The model under review builds one solid part; all positions refer to its coordinate system, in mm. Face numbers are marked on the shaded views. A direction names the side the tool comes from. Coordinates: 2 decimals unless noted, no trailing zeros. Order: outer loops, then holes, each group sorted by start corner. A loop starts at its lowest first (then second) coordinate and runs counter-clockwise, first axis right, second up. Notation, with made-up numbers: M 9,58.5 L 66,58.5 A31 ccw 66,93.5 Z; hole C -14,25 d8. An arc over 180 degrees is marked long. Answer in a Markdown table with one row per item.
Autodesk Inventor part; units mm, degrees
ref_plane "YZ Plane" through (0, 0, 0) normal (1, 0, 0) x (0, 1, 0)
ref_plane "XZ Plane" through (0, 0, 0) normal (0, 1, 0) x (-1, 0, 0)
ref_plane "XY Plane" through (0, 0, 0) normal (0, 0, 1) x (1, 0, 0)
sketch "Sketch2" plane through (0, 0, 0) normal (0, 1, 0) x (-1, 0, 0)
  line L0 (0, 0) -> (0, -12)
  line L1 (0, 0) -> (0, 10)
  line L2 (0, -12) -> (-2, -12)
  line L3 (-2, -12) -> (-2, -4)
  line L4 (-3, -4) -> (-2, -4)
  line L5 (-3, -4) -> (-3, -2.5) construction
  line L6 (-2, 10) -> (0, 10)
  line L7 (-3, -2.5) -> (0, -2.5) construction
  circle A0 centre (-1.2, -2.5) radius 0.95
  line L8 (-3, -4) -> (-3, 10)
  line L9 (-3, 10) -> (-2, 10)
  line L10 (0, 0) -> (-3, 0) construction
  dimension "d1" = 10
  dimension "d2" = 2
  dimension "d9" = 1.9
  dimension "d10" = 8
  dimension "d11" = 3
  dimension "d12" = 1.8
  dimension "d38" = 4
extrude "Extrusion1" add sketch "Sketch2" along normal blind 3.5
sketch "Sketch3" plane through (3, 0, 10) normal (1, 0, 0) x (0, 0, -1)
  line L0 (0, 0) -> (0, 3.5)
  line L1 (0, 1.75) -> (22, 1.75) construction
  line L2 (22, 1.75) -> (22, 2.15)
  line L3 (22, 0) -> (22, 3.5)
  line L4 (11, 2.15) -> (11, 1.35)
  line L5 (22, 2.15) -> (21.1843, 2.15)
  line L6 (18.8157, 2.15) -> (11, 2.15)
  line L7 (11, 1.35) -> (18.8157, 1.35)
  line L8 (21.1843, 1.35) -> (22, 1.35)
  arc A0 (18.8157, 1.35) -> (21.1843, 1.35) centre (20, 1.75) ccw
  arc A1 (21.1843, 2.15) -> (18.8157, 2.15) centre (20, 1.75) ccw
  line L9 (22, 1.75) -> (22, 1.35)
  point P0 (10, 0)
  dimension "d16" = 2
  dimension "d17" = 0.4
  dimension "d18" = 11
  dimension "d19" = 0.8
extrude "Extrusion2" cut sketch "Sketch3" against normal blind 10
sketch "Sketch4" plane through (0, 0, -12) normal (-1, 0, 0) x (0, 0, 1)
  point P0 (12, 0)
sketch "Sketch5" plane through (0, 0, -12) normal (-1, 0, 0) x (0, 0, 1)
  line L0 (16, 0) -> (16, -1)
  line L1 (16, -1) -> (22, -1)
  line L2 (22, 0) -> (16, 0)
  line L3 (16, 3.5) -> (16, 4.5)
  line L4 (16, 4.5) -> (22, 4.5)
  line L5 (22, 3.5) -> (16, 3.5)
  line L6 (22, 4.5) -> (27, 4.5)
  line L7 (27, 4.5) -> (27, -1)
  line L8 (27, -1) -> (22, -1)
  line L9 (22, 3.5) -> (22, 0)
  line L10 (12, 0) -> (12, 3.5) construction
  dimension "d23" = 1
  dimension "d24" = 1
  dimension "d27" = 5
  dimension "d39" = 5.5
  dimension "d40" = 4
extrude "Extrusion3" add sketch "Sketch5" against normal blind 3
sketch "Sketch6" plane through (0, 0, -12) normal (-1, 0, 0) x (0, 0, 1)
  line L0 (22, 1.75) -> (14, 1.75) construction
  line L1 (27, 4.5) -> (16, 4.5)
  circle A0 centre (24.5, 1.75) radius 0.95
  line L2 (27, -1) -> (27, 4.5)
  circle A1 centre (18.5, 1.75) radius 0.95
  point P0 (12, 0)
  dimension "d28" = 2.75
  dimension "d32" = 1.9
  dimension "d33" = 2.5
  dimension "d34" = 1.9
  dimension "d35" = 6
extrude "Extrusion4" cut sketch "Sketch6" against normal blind 3
properties part number "ferrule holder"
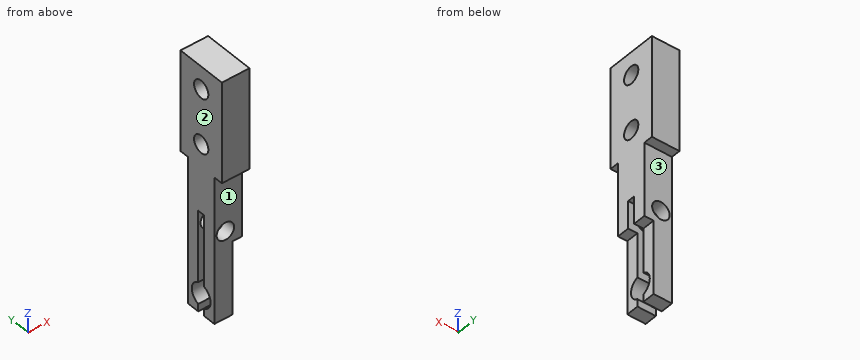
(1) Take a section at C-C (x = 2.6). Write out the cut boundary in (y, z), then the cut area to 3 significant figures.
Report:
| item | result |
|---|---|
| outline | M -1,4 L 0,4 L 0,-4 L 1.35,-4 L 1.35,-1 L 2.15,-1 L 2.15,-4 L 3.5,-4 L 3.5,4 L 4.5,4 L 4.5,15 L -1,15 Z; hole C 1.75,6.5 d1.9; hole C 1.75,12.5 d1.9 |
| area | 80.4 mm^2 |
(2) Take a section at A-A (x = 1.2). Write out the cut boundary in (y, z).
Report:
| item | result |
|---|---|
| outline | M -1,4 L 0,4 L 0,-1.55 L 1.35,-1.55 L 1.35,-1 L 2.15,-1 L 2.15,-1.55 L 3.5,-1.55 L 3.5,4 L 4.5,4 L 4.5,15 L -1,15 Z; M 0,-12 L 1.35,-12 L 1.35,-11.18 A1.25 cw 1.35,-8.82 L 1.35,-3.45 L 0,-3.45 Z; M 2.15,-12 L 3.5,-12 L 3.5,-3.45 L 2.15,-3.45 L 2.15,-8.82 A1.25 cw 2.15,-11.18 Z; hole C 1.75,6.5 d1.9; hole C 1.75,12.5 d1.9 |
(3) Take a section at B-B (z = -2.5). Write out the cut boundary in (x, y).
Report:
| item | result |
|---|---|
| outline | M 0,0 L 0.25,0 L 0.25,1.35 L 0,1.35 Z; M 0,2.15 L 0.25,2.15 L 0.25,3.5 L 0,3.5 Z; M 2.15,0 L 3,0 L 3,1.35 L 2.15,1.35 Z; M 2.15,2.15 L 3,2.15 L 3,3.5 L 2.15,3.5 Z |
(4) To check wall thickness, follow line 1 (Y direction, x = 0.8, z = 12.5); line 2 (Z direction, x = 1.2, y = 2.8); line 3 (Z direction, x = 1.9, y = 2.5). State the ranges of each line that lie inside material, in increasing order. Write a range as [from, to].
Report:
| item | result |
|---|---|
| line 1 | [-1, 0.8], [2.7, 4.5] |
| line 2 | [-12, -10.68], [-9.32, -3.45], [-1.55, 15] |
| line 3 | [-12, -11], [-9, -3.14], [-1.86, 5.92], [7.08, 11.92], [13.08, 15] |
(5) Take a section at D-D (y = 1.75). Write out the cut boundary in (x, z).
Report:
| item | result |
|---|---|
| outline | M 0,-1 L 3,-1 L 3,5.55 L 0,5.55 Z; M 0,7.45 L 3,7.45 L 3,11.55 L 0,11.55 Z; M 0,13.45 L 3,13.45 L 3,15 L 0,15 Z |
(6) Insertion check: P1, Ø0.5, axis at x = 1, y = 4, coming from the -Z side; P2, Ø0.9, axis at x = 1, z = -11.5, coming from the +Y side; P3, Ø0.7, axis at y = 3, z = -7.5, coming from the +X side. Each pin has a flat end and moves straight along its axis. Give the tip position at first contact, or say it passes through.
Report:
| item | result |
|---|---|
| P1 | z = 4 |
| P2 | y = 3.5 |
| P3 | x = 2 |
(7) Machinability: for the marked faces 1, 2 and 3, which of the approach directions +Z, -Z, +X, -X, +Y, -Y give a long, thin tool a straight path to every point of the face, cutting with its end or side? Answer none if there is none.
Report:
| item | result |
|---|---|
| face 1 | -Z, +X, -X, -Y |
| face 2 | +Z, -Z, -X, +Y, -Y |
| face 3 | -Z, +X, -X, +Y |
